Geometry check sheet. Reference: the model listing, model coordinates, mm. Round coordinates to 2 decimals unless told otherwise and drop trailing zeros. Write each loop counter-clockwise with the first axis right and the second up, starting at its lowest first coordinate (ties: lowest second). Pieces come first, ordered by that corner, then holes. Notation, with made-up numbers: M 46,-37 L 97,-37 A22 cw 97,-9 Z; hole C 54.25,43.5 d3. An arc over 180 degrees is marked long. Use a Markdown table: item, result.
```python
from build123d import *

# Parameters (mm, degrees)
ESQUISSE2_W             = 40
ESQUISSE2_H             = 10
BOSS_EXTRU_2_DEPTH      = 13.5
ENL_V_MAT_EXTRU_3_DEPTH = 30.780378473
ESQUISSE5_R             = 2
ENL_V_MAT_EXTRU_4_DEPTH = 32.649869703


with BuildPart() as part:
    # Esquisse2 → Boss.-Extru.2 (new body)
    with BuildSketch(Plane(origin=(0, 0, 0), x_dir=(1, 0, 0), z_dir=(0, 1, 0))):
        with Locations((4.589041096, 9.657534247)):
            Rectangle(ESQUISSE2_W, ESQUISSE2_H)
    extrude(amount=BOSS_EXTRU_2_DEPTH)

    # Esquisse4 → Enlèv. mat.-Extru.3 (cut, through all)
    with BuildSketch(Plane.XY.offset(-4.657534247)):
        with BuildLine():
            Line((-6.399589392, 0), (15.577671584, 0))
            ThreePointArc((15.577671584, 0), (4.589041096, 10.5), (-6.399589392, 0))
        make_face()
    extrude(amount=-ENL_V_MAT_EXTRU_3_DEPTH, mode=Mode.SUBTRACT)

    # Esquisse5 → Enlèv. mat.-Extru.4 (cut, through all)
    with BuildSketch(Plane(origin=(0, 13.5, 0), x_dir=(1, 0, 0), z_dir=(0, 1, 0))):
        with Locations(Location((-10.910958904, 9.657534247, 0), (0, 0, 270))):
            Circle(ESQUISSE5_R)
        with Locations(Location((20.089041096, 9.657534247, 0), (0, 0, 90))):
            Circle(ESQUISSE5_R)
    extrude(amount=-ENL_V_MAT_EXTRU_4_DEPTH, mode=Mode.SUBTRACT)


solid = part.part
```
Item 1: Cross-section at C-C, the plane x = 19. Record the cut outline in (y, z), and give its area (3 significant figures).
Outcome:
| item | result |
|---|---|
| outline | M 0,-14.66 L 13.5,-14.66 L 13.5,-11.34 L 0,-11.34 Z; M 0,-7.98 L 13.5,-7.98 L 13.5,-4.66 L 0,-4.66 Z |
| area | 89.7 mm2 |
Item 2: Cross-section at B-B, the plane z = -9.75. Record the cut outline in (x, y), and give its area (3 significant figures).
Outcome:
| item | result |
|---|---|
| outline | M -15.41,0 L -12.91,0 L -12.91,13.5 L -15.41,13.5 Z; M -8.91,0 L -6.4,0 A11 cw 15.58,0 L 18.09,0 L 18.09,13.5 L -8.91,13.5 Z; M 22.09,0 L 24.59,0 L 24.59,13.5 L 22.09,13.5 Z |
| area | 253 mm2 |
Item 3: Go/stop test with a flat-tipped pin: pin 1 (6 mm diameter, centred on x = 11, z = -12, fed in from -Y). Record where the tip stops, or that it passes through.
Outcome:
| item | result |
|---|---|
| pin 1 | stops at y = 5.2 |
Item 4: Cross-section at A-A, the plane y = 8.5. Record the cut outline in (x, z), and give its area (3 significant figures).
Outcome:
| item | result |
|---|---|
| outline | M -15.41,-14.66 L -1.74,-14.66 L -1.74,-4.66 L -15.41,-4.66 Z; M 10.91,-14.66 L 24.59,-14.66 L 24.59,-4.66 L 10.91,-4.66 Z; hole C -10.91,-9.66 d4; hole C 20.09,-9.66 d4 |
| area | 248 mm2 |
Item 5: Mould release check, pull along Z, two halves, no side actions. Record for faces 1 (the face through (21.863, 6.844, -10.58)), 2 (the face through (4, 11, -4.658)), 3 (the face through (4.824, 10.497, -9.588)): +Z half, -Z half, draft (parallel to the pull), parting line (faces both ways), or undercut.
Outcome:
| item | result |
|---|---|
| face 1 | undercut |
| face 2 | +Z half |
| face 3 | draft |
Item 6: Cross-section at D-D, the plane y = 4.25. Record the cut outline in (x, z), and give its area (3 significant figures).
Outcome:
| item | result |
|---|---|
| outline | M -15.41,-14.66 L -5.33,-14.66 L -5.33,-4.66 L -15.41,-4.66 Z; M 14.51,-14.66 L 24.59,-14.66 L 24.59,-4.66 L 14.51,-4.66 Z; hole C -10.91,-9.66 d4; hole C 20.09,-9.66 d4 |
| area | 176 mm2 |
Item 7: Material ranges on line 1 along X through (y, z) = (8.25, -7); line 2 along X through (y, z) = (7.25, -10.25); line 3 along X through (y, z) = (9, -9), recorded low to high. Write a range as from..to.
Outcome:
| item | result |
|---|---|
| line 1 | x = -15.41..-2.08, 11.26..24.59 |
| line 2 | x = -15.41..-12.82, -9..-3.22, 12.4..18.18, 22..24.59 |
| line 3 | x = -15.41..-12.8, -9.02..-0.96, 10.13..18.2, 21.98..24.59 |
